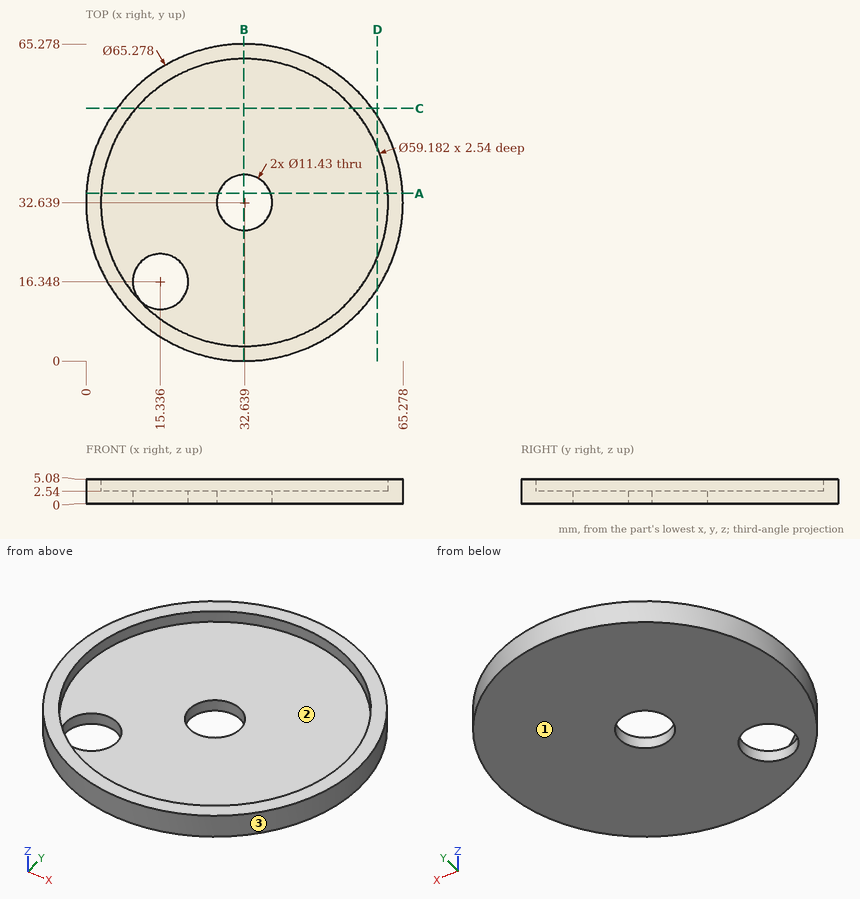
Geometry check sheet. Reference: drawing and pictorial views, mm from the part's lowest x, y, z. Give positions to 0.01 mm unless a question says otherwise; leave off trailing zeros. Write each loop counter-clockwise with the first axis right and the second up, starting at its lowest first coordinate (ties: lowest second). Pieces come first, ordered by that corner, then holes. Notation, with made-up numbers: (61, -9.75) -> (71, -9.75) arc R24 ccw to (71, 15.25) -> close; hole circle Ø2 at (88.5, 61.25). An arc over 180 degrees is marked (long way). One line per question, with ' | ' between items.
Item 1: Sectioned sample at D-D, the plane x = 60. Record the boundary of the cut face in (y, z).
Determined:
outline: (14.84, 0) -> (50.43, 0) -> (50.43, 5.08) -> (43.91, 5.08) -> (43.91, 2.54) -> (21.37, 2.54) -> (21.37, 5.08) -> (14.84, 5.08) -> close
Item 2: Depth check by flat-ended pin: pin 1 (8 mm diameter, centred on x = 11, y = 29.5, fed in from +Z); pin 2 (2 mm diameter, centred on x = 53.5, z = 1.5, fed in from +Y); pin 3 (10.5 mm diameter, centred on x = 32.639, y = 32.639, fed in from +Z); pin 4 (3 mm diameter, centred on x = 16, z = 1, fed in from +Y) (1 decimal). Enter the tip coordinate at first touch or a pass-through.
Determined:
pin 1: z = 2.54 | pin 2: y = 58.54 | pin 3: through | pin 4: y = 61.6
Item 3: Sectioned sample at B-B, the plane x = 32.5. Record the boundary of the cut face in (y, z), plus the area to 3 significant figures.
Determined:
outline: (0, 0) -> (26.93, 0) -> (26.93, 2.54) -> (3.05, 2.54) -> (3.05, 5.08) -> (0, 5.08) -> close; (38.35, 0) -> (65.28, 0) -> (65.28, 5.08) -> (62.23, 5.08) -> (62.23, 2.54) -> (38.35, 2.54) -> close | area: 152 mm^2
Item 4: Scan lines: line 1 along Z through (x, y) = (32, 41.5); line 2 along X through (y, z) = (30, 3.4); line 3 along X through (y, z) = (9, 4.6) (1 decimal). Record each from-to range of solid material in increasing order.
Determined:
line 1: 0 to 2.54 | line 2: 0.11 to 3.17, 62.11 to 65.17 | line 3: 10.1 to 14.8, 50.4 to 55.1
Item 5: Draft check along X on the marked faces 1, 2 and 3. Enter one of: released by +X, released by -X, zero draft, split by the parting line, or undercut.
Determined:
face 1: zero draft | face 2: undercut | face 3: split by the parting line
Item 6: Sectioned sample at A-A, the plane y = 34.5. Record the boundary of the cut face in (x, z) (1 decimal), plus the area to 3 significant figures.
Determined:
outline: (0.1, 0) -> (27.2, 0) -> (27.2, 2.5) -> (3.1, 2.5) -> (3.1, 5.1) -> (0.1, 5.1) -> close; (38, 0) -> (65.2, 0) -> (65.2, 5.1) -> (62.2, 5.1) -> (62.2, 2.5) -> (38, 2.5) -> close | area: 154 mm^2
Item 7: Sectioned sample at C-C, the plane y = 52. Record the boundary of the cut face in (x, z).
Determined:
outline: (6.36, 0) -> (58.92, 0) -> (58.92, 5.08) -> (55.02, 5.08) -> (55.02, 2.54) -> (10.26, 2.54) -> (10.26, 5.08) -> (6.36, 5.08) -> close
